Source: CAD feature listing. Evaluate the final solid. Frame: model axes, mm. A direction names the side the tool comes from. Give positions to 0.01 mm unless a question says otherwise; leave off trailing zeros. Order: outer loops, then holes, each group sorted by start corner. A loop starts at its lowest first (then second) coordinate and runs counter-clockwise, first axis right, second up. Notation, with made-up numbers: M -37.75,29 L 21.25,29 A20 cw 21.25,43 Z; hole C 12,57 d10. An arc over 180 degrees is marked long. Answer in a Markdown table with one row per item. Add a question column.
(1) Pin query (flat end, axial travel): P1, Ø0.9, axis at x = 13.44, z = 11.31, coming from the -Y side; P2, Ø1.2, axis at x = -0.5, y = -1.5, coming from the +Z side; P3, Ø1.2, axis at y = -2, z = -0.5, coming from the +X side; P4, Ø0.9, axis at y = -2, z = -21, coming from the +X side. Return the tip coordinate at first contact, or that it passes through.
(2) Mould query, pull axis Z, two halves, no side actions, for faces 1 (the face through (-16.37, -1.48, -14.25)), 2 (the face through (23.14, -1.48, 9.46)), 3 (the face through (-1.5, -1, -22)). Classes: pulls with the +Z half, pulls with the -Z half, needs draft (parallel to the pull), parting line crosses it, or undercut.
(3) Material intervals for line 1 along Z through (x, y) = (16, -1.4); line 2 along X through (y, z) = (-0.05, 13); line 3 along Z through (x, y) = (14.5, -0.5), sorted ascending.
(4) Section query A-A, the plane x = -4. Return loops of the section in (y, z), plus the area to 3 significant figures.
(5) Section query B-B, the plane x = 3.5. Return loops of the section in (y, z), plus the area to 3 significant figures.
(6) Set-up query: faces 4 (the face through (-17.5, -1, 0)), 5 (the face through (22, -1, 1.5)), 6 (the face through (-14.18, -1.48, -16.3)), 7 (the face through (-1.5, -1, 22)). Return all of +Z, -Z, +X, -X, +Y, -Y with unobstructed straight access to the full face (end or side cutting, diameter ignored); none if empty.
from build123d import *

# Parameters (mm, degrees)
F2_DEPTH = 3


with BuildPart() as f2:
    # F1 (on Front) → F2 (new body)
    with BuildSketch(Plane.XZ):
        with BuildLine():
            Line((18.25, 1.5), (24.9549594269, 1.5))
            ThreePointArc((24.9549594269, 1.5), (23.0969883128, 9.5670858091), (18.7064812068, 16.5851608632))
            Line((18.7064812068, 16.5851608632), (13.9653589284, 11.8440385849))
            ThreePointArc((13.9653589284, 11.8440385849), (14.1279384919, 11.6007210733), (14.1850288425, 11.313708499))
            ThreePointArc((14.1850288425, 11.313708499), (13.1480162683, 10.6207988496), (12.9046987567, 11.8440385849))
            Line((12.9046987567, 11.8440385849), (11.8440385849, 12.9046987567))
            ThreePointArc((11.8440385849, 12.9046987567), (10.563708499, 13.4350288425), (11.8440385849, 13.9653589284))
            Line((11.8440385849, 13.9653589284), (16.5851608632, 18.7064812068))
            ThreePointArc((16.5851608632, 18.7064812068), (9.5670858091, 23.0969883128), (1.5, 24.9549594269))
            Line((1.5, 24.9549594269), (1.5, 18.25))
            ThreePointArc((1.5, 18.25), (2.0303300859, 18.0303300859), (2.25, 17.5))
            ThreePointArc((2.25, 17.5), (1.5, 16.75), (0.75, 17.5))
            Line((0.75, 17.5), (-0.75, 17.5))
            ThreePointArc((-0.75, 17.5), (-2.0303300859, 16.9696699141), (-1.5, 18.25))
            Line((-1.5, 18.25), (-1.5, 24.9549594269))
            ThreePointArc((-1.5, 24.9549594269), (-9.5670858091, 23.0969883128), (-16.5851608632, 18.7064812068))
            Line((-16.5851608632, 18.7064812068), (-11.8440385849, 13.9653589284))
            ThreePointArc((-11.8440385849, 13.9653589284), (-11.0266959247, 14.1279384919), (-10.563708499, 13.4350288425))
            ThreePointArc((-10.563708499, 13.4350288425), (-11.0266959247, 12.7421191932), (-11.8440385849, 12.9046987567))
            Line((-11.8440385849, 12.9046987567), (-12.9046987567, 11.8440385849))
            ThreePointArc((-12.9046987567, 11.8440385849), (-12.7421191932, 11.6007210733), (-12.6850288425, 11.313708499))
            ThreePointArc((-12.6850288425, 11.313708499), (-13.7220414168, 10.6207988496), (-13.9653589284, 11.8440385849))
            Line((-13.9653589284, 11.8440385849), (-18.7064812068, 16.5851608632))
            ThreePointArc((-18.7064812068, 16.5851608632), (-23.0969883128, 9.5670858091), (-24.9549594269, 1.5))
            Line((-24.9549594269, 1.5), (-18.25, 1.5))
            ThreePointArc((-18.25, 1.5), (-17.5, 2.25), (-16.75, 1.5))
            ThreePointArc((-16.75, 1.5), (-16.9696699141, 0.9696699141), (-17.5, 0.75))
            Line((-17.5, 0.75), (-17.5, -0.75))
            ThreePointArc((-17.5, -0.75), (-16.9696699141, -0.9696699141), (-16.75, -1.5))
            ThreePointArc((-16.75, -1.5), (-17.5, -2.25), (-18.25, -1.5))
            Line((-18.25, -1.5), (-24.9549594269, -1.5))
            ThreePointArc((-24.9549594269, -1.5), (-23.0969883128, -9.5670858091), (-18.7064812068, -16.5851608632))
            Line((-18.7064812068, -16.5851608632), (-13.9653589284, -11.8440385849))
            ThreePointArc((-13.9653589284, -11.8440385849), (-13.7220414168, -10.6207988496), (-12.6850288425, -11.313708499))
            ThreePointArc((-12.6850288425, -11.313708499), (-12.7421191932, -11.6007210733), (-12.9046987567, -11.8440385849))
            Line((-12.9046987567, -11.8440385849), (-11.8440385849, -12.9046987567))
            ThreePointArc((-11.8440385849, -12.9046987567), (-11.0266959247, -12.7421191932), (-10.563708499, -13.4350288425))
            ThreePointArc((-10.563708499, -13.4350288425), (-11.0266959247, -14.1279384919), (-11.8440385849, -13.9653589284))
            Line((-11.8440385849, -13.9653589284), (-16.5851608632, -18.7064812068))
            ThreePointArc((-16.5851608632, -18.7064812068), (-9.5670858091, -23.0969883128), (-1.5, -24.9549594269))
            Line((-1.5, -24.9549594269), (-1.5, -18.25))
            ThreePointArc((-1.5, -18.25), (-2.0303300859, -16.9696699141), (-0.75, -17.5))
            Line((-0.75, -17.5), (0.75, -17.5))
            ThreePointArc((0.75, -17.5), (1.5, -16.75), (2.25, -17.5))
            ThreePointArc((2.25, -17.5), (2.0303300859, -18.0303300859), (1.5, -18.25))
            Line((1.5, -18.25), (1.5, -24.9549594269))
            ThreePointArc((1.5, -24.9549594269), (9.5670858091, -23.0969883128), (16.5851608632, -18.7064812068))
            Line((16.5851608632, -18.7064812068), (11.8440385849, -13.9653589284))
            ThreePointArc((11.8440385849, -13.9653589284), (10.563708499, -13.4350288425), (11.8440385849, -12.9046987567))
            Line((11.8440385849, -12.9046987567), (12.9046987567, -11.8440385849))
            ThreePointArc((12.9046987567, -11.8440385849), (13.1480162683, -10.6207988496), (14.1850288425, -11.313708499))
            ThreePointArc((14.1850288425, -11.313708499), (14.1279384919, -11.6007210733), (13.9653589284, -11.8440385849))
            Line((13.9653589284, -11.8440385849), (18.7064812068, -16.5851608632))
            ThreePointArc((18.7064812068, -16.5851608632), (23.0969883128, -9.5670858091), (24.9549594269, -1.5))
            Line((24.9549594269, -1.5), (18.25, -1.5))
            ThreePointArc((18.25, -1.5), (16.9696699141, -2.0303300859), (17.5, -0.75))
            Line((17.5, -0.75), (17.5, 0.75))
            ThreePointArc((17.5, 0.75), (16.9696699141, 2.0303300859), (18.25, 1.5))
        make_face()
        with BuildLine():
            ThreePointArc((9.8767656083, 1.5650882145), (9.9691437968, 0.7849662149), (10, 0))
            ThreePointArc((10, 0), (9.9338326925, -1.1484633378), (9.7362063924, -2.2817285302))
            ThreePointArc((9.7362063924, -2.2817285302), (10.7093913456, -3.0062809605), (11.0798284208, -4.1616343917))
            ThreePointArc((11.0798284208, -4.1616343917), (10.081943125, -5.884910827), (8.0906124274, -5.8772434482))
            ThreePointArc((8.0906124274, -5.8772434482), (6.8081540818, -7.3245503615), (5.2711118466, -8.4979632796))
            ThreePointArc((5.2711118466, -8.4979632796), (5.4225096089, -8.9235676616), (5.4738602751, -9.3723699359))
            ThreePointArc((5.4738602751, -9.3723699359), (3.7412190824, -11.3429608382), (1.5650882145, -9.8767656083))
            ThreePointArc((1.5650882145, -9.8767656083), (-0.3651473111, -9.9933311484), (-2.2817285302, -9.7362063924))
            ThreePointArc((-2.2817285302, -9.7362063924), (-4.9885220711, -10.8995936469), (-5.8772434482, -8.0906124274))
            ThreePointArc((-5.8772434482, -8.0906124274), (-7.3245503615, -6.8081540818), (-8.4979632796, -5.2711118466))
            ThreePointArc((-8.4979632796, -5.2711118466), (-11.2345943645, -4.1797587953), (-9.8767656083, -1.5650882145))
            ThreePointArc((-9.8767656083, -1.5650882145), (-9.9933311484, 0.3651473111), (-9.7362063924, 2.2817285302))
            ThreePointArc((-9.7362063924, 2.2817285302), (-10.8995936469, 4.9885220711), (-8.0906124274, 5.8772434482))
            ThreePointArc((-8.0906124274, 5.8772434482), (-6.8081540818, 7.3245503615), (-5.2711118466, 8.4979632796))
            ThreePointArc((-5.2711118466, 8.4979632796), (-4.1797587953, 11.2345943645), (-1.5650882145, 9.8767656083))
            ThreePointArc((-1.5650882145, 9.8767656083), (0.3651473111, 9.9933311484), (2.2817285302, 9.7362063924))
            ThreePointArc((2.2817285302, 9.7362063924), (4.487709352, 11.0528897352), (6.1485645292, 9.0928982833))
            ThreePointArc((6.1485645292, 9.0928982833), (6.0795351595, 8.5737181445), (5.8772434482, 8.0906124274))
            ThreePointArc((5.8772434482, 8.0906124274), (7.3245503615, 6.8081540818), (8.4979632796, 5.2711118466))
            ThreePointArc((8.4979632796, 5.2711118466), (10.423680174, 5.1729426389), (11.3593000735, 3.4869301375))
            ThreePointArc((11.3593000735, 3.4869301375), (10.9455975631, 2.2733213849), (9.8767656083, 1.5650882145))
        make_face(mode=Mode.SUBTRACT)
    extrude(amount=F2_DEPTH)


solid = f2.part
Values follow:
| question | item | result |
|---|---|---|
| 1 | P1 | passes through |
| 1 | P2 | stops at z = 17.5 |
| 1 | P3 | stops at x = 17.5 |
| 1 | P4 | stops at x = 14.24 |
| 2 | face 1 | undercut |
| 2 | face 2 | pulls with the +Z half |
| 2 | face 3 | needs draft |
| 3 | line 1 | z = -19.21 to -18.12, -13.88 to 13.88, 18.12 to 19.21 |
| 3 | line 2 | x = -21.35 to -15.12, -10.7 to 10.7, 15.12 to 21.35 |
| 3 | line 3 | z = -20.37 to -16.62, -12.38 to 12.38, 16.62 to 20.37 |
| 4 | outline | M -3,-24.68 L 0,-24.68 L 0,-11.07 L -3,-11.07 Z; M -3,11.29 L 0,11.29 L 0,24.68 L -3,24.68 Z |
| 4 | area | 81.0 mm² |
| 5 | outline | M -3,-24.75 L 0,-24.75 L 0,-11.36 L -3,-11.36 Z; M -3,10.97 L 0,10.97 L 0,24.75 L -3,24.75 Z |
| 5 | area | 81.5 mm² |
| 6 | face 4 | -X, +Y, -Y |
| 6 | face 5 | +X, +Y, -Y |
| 6 | face 6 | +Y, -Y |
| 6 | face 7 | +Z, +Y, -Y |
